Design review of the part built by this model. Coordinates are the model's own, in mm. A direction names the side the tool comes from. Round coordinates to 2 decimals unless told otherwise and drop trailing zeros. Loops run counter-clockwise (first coordinate to the right, second up) from the corner with the lowest first, then second, coordinate; pieces in that order, holes last. Notation, with made-up numbers: M 55,-25 L 86,-25 A31 ccw 86,5 Z; hole C 85,36.25 d11. An arc over 180 degrees is marked long. Use a Markdown table: item, result.
from build123d import *

# Parameters (mm, degrees)
F0_W     = 54.3052
F0_H     = 113.3856
F0_R     = 12.0015
F1_DEPTH = 2.4638
F0_W_2   = 62.611
F0_H_2   = 121.6914
F2_DEPTH = 11.8364
F3_W     = 47.5488
F3_H     = 5.9055
F4_DEPTH = 25.4


with BuildPart() as f1:
    # F0 (on Front) → F1 (new body)
    with BuildSketch(Plane.XZ):
        Rectangle(F0_W, F0_H)
        with Locations((0, 29.2735)):
            Circle(F0_R, mode=Mode.SUBTRACT)
        with BuildLine():
            ThreePointArc((16.0909, 42.672), (9.2964, 49.4665), (16.0909, 56.261))
            Line((16.0909, 56.261), (20.066003, 56.261))
            ThreePointArc((20.066003, 56.261), (26.8605, 49.466498), (20.066, 42.672))
            Line((20.066, 42.672), (16.0909, 42.672))
        make_face(mode=Mode.SUBTRACT)
    extrude(amount=F1_DEPTH)

    # F0 (on Front) → F2 (join)
    with BuildSketch(Plane.XZ):
        Rectangle(F0_W_2, F0_H_2)
        Rectangle(F0_W, F0_H, mode=Mode.SUBTRACT)
    extrude(amount=F2_DEPTH)

    # F3 (on face) → F4 (cut)
    with BuildSketch(Plane(origin=(0, 0, -60.8457), x_dir=(1, 0, 0), z_dir=(0, 0, -1))):
        with Locations((0, 5.28955)):
            Rectangle(F3_W, F3_H)
    extrude(amount=-F4_DEPTH, mode=Mode.SUBTRACT)


solid = f1.part
1. Take a section at D-D on x = 0. Give the boundary of the cut face in (y, z) (3 decimals), and give its area (3 significant figures).
Check values:
| item | result |
|---|---|
| outline | M -11.836,-60.846 L -8.242,-60.846 L -8.242,-56.693 L -11.836,-56.693 Z; M -11.836,56.693 L -2.464,56.693 L -2.464,41.275 L 0,41.275 L 0,60.846 L -11.836,60.846 Z; M -2.464,-35.446 L -2.337,-35.446 L -2.337,-60.846 L 0,-60.846 L 0,17.272 L -2.464,17.272 Z |
| area | 291 mm² |
2. Insertion check: pin 1 (4 mm diameter, centred on x = 12, z = 32.5, fed in from +Y); pin 2 (1 mm diameter, centred on x = -15, z = 11.5, fed in from -Y); pin 3 (12.5 mm diameter, centred on x = -2, z = -47.5, fed in from -Y). Each pin has a flat end and moves straight along its axis. Give the tip position at first contact, or say it passes through.
Check values:
| item | result |
|---|---|
| pin 1 | stops at y = 0 |
| pin 2 | stops at y = -2.46 |
| pin 3 | stops at y = -2.34 |
3. Take a section at A-A on x = 17.5. Give the boundary of the cut face in (y, z).
Check values:
| item | result |
|---|---|
| outline | M -11.84,-60.85 L -8.24,-60.85 L -8.24,-56.69 L -11.84,-56.69 Z; M -11.84,56.69 L -2.46,56.69 L -2.46,56.26 L 0,56.26 L 0,60.85 L -11.84,60.85 Z; M -2.46,-35.45 L -2.34,-35.45 L -2.34,-60.85 L 0,-60.85 L 0,42.67 L -2.46,42.67 Z |
4. Machinability: for faces 1 (the face through (18, -1, 42.672)), 2 (the face through (-23.774, -5, -58)), 3 (the face through (27.153, -7, -1)), 4 (the face through (-28, -11.836, 5)), which of the approach directions +Z, -Z, +X, -X, +Y, -Y give a long, thin tool a straight path to every point of the face, cutting with its end or side? Answer none if there is none.
Check values:
| item | result |
|---|---|
| face 1 | +Y, -Y |
| face 2 | -Z |
| face 3 | -Y |
| face 4 | +Z, -Z, +X, -X, -Y |
5. Take a section at C-C on z = -15. Give the boundary of the cut face in (x, y).
Check values:
| item | result |
|---|---|
| outline | M -31.31,-11.84 L -27.15,-11.84 L -27.15,-2.46 L 27.15,-2.46 L 27.15,-11.84 L 31.31,-11.84 L 31.31,0 L -31.31,0 Z |
6. Wall thickness on line 1 along X through (y, z) = (-10.5, 50.5); line 2 along Z through (x, y) = (-8, -10.25); line 3 along Z through (x, y) = (0, -1.45) (3 decimals): over which ranges is each line inside the solid? List them lowest first. Write a range as from..to.
Check values:
| item | result |
|---|---|
| line 1 | x = -31.31..-27.15, 27.15..31.31 |
| line 2 | z = -60.85..-56.69, 56.69..60.85 |
| line 3 | z = -60.846..17.272, 41.275..60.846 |
7. The part is to be moulded in two halves that separate along Y. For faces 5 (the face through (0, -2.464, 13)), 6 (the face through (26.86, -1.21, 49.62)), 7 (the face through (0, -2.337, -48)), say which applies: pulls with the +Y half, pulls with the -Y half, needs draft (parallel to the pull), parting line crosses it, or undercut.
Check values:
| item | result |
|---|---|
| face 5 | pulls with the -Y half |
| face 6 | needs draft |
| face 7 | undercut |
8. Take a section at B-B on y = -10. Give the boundary of the cut face in (x, z), and give its area (3 significant figures).
Check values:
| item | result |
|---|---|
| outline | M -31.31,-60.85 L 31.31,-60.85 L 31.31,60.85 L -31.31,60.85 Z; hole M -27.15,-56.69 L 27.15,-56.69 L 27.15,56.69 L -27.15,56.69 Z |
| area | 1,460 mm² |
